Check sheet for the modelled part. Datum: model origin and axes. Units: mm. A direction names the side the tool comes from. Round coordinates to 2 decimals unless told otherwise and drop trailing zeros. Loops run counter-clockwise (first coordinate to the right, second up) from the corner with the lowest first, then second, coordinate; pieces in that order, holes last. Notation, with made-up numbers: (25.5, 3.5) - (49.5, 3.5) arc R19 cw to (49.5, 31.5) - close; hole circle Ø9 at (54.25, 19). An arc over 180 degrees is marked (long way). Put each result on its own line as item: value. Start each with the question number.
```python
from build123d import *

# Parameters (mm, degrees)
BOX001_W          = 50
BOX001_H          = 44
BOX001_DEPTH      = 12.7
CYLINDER001_R     = 6.223
CYLINDER001_DEPTH = 19.05
CYLINDER_R        = 3.175
CYLINDER_DEPTH    = 25.4
CYLINDER003_R     = 6.223
CYLINDER003_DEPTH = 19.05
CYLINDER002_R     = 3.175
CYLINDER002_DEPTH = 25.4
CYLINDER005_R     = 6.223
CYLINDER005_DEPTH = 19.05
CYLINDER004_R     = 3.175
CYLINDER004_DEPTH = 25.4
BOX_W             = 50
BOX_H             = 44
BOX_DEPTH         = 12.7


with BuildPart() as top_plate:
    # Box001 → Box001 (new body)
    with BuildSketch(Plane.XY.offset(21)):
        with Locations((25, 22)):
            Rectangle(BOX001_W, BOX001_H)
    extrude(amount=BOX001_DEPTH)


with BuildPart() as screw_cap:
    # Cylinder001 → Cylinder001 (new body)
    with BuildSketch(Plane.XY.offset(25.4)):
        Circle(CYLINDER001_R)
    extrude(amount=CYLINDER001_DEPTH)


with BuildPart() as left_screw:
    # Cylinder → Cylinder (new body)
    with BuildSketch(Plane.XY):
        Circle(CYLINDER_R)
    extrude(amount=CYLINDER_DEPTH)

    # Fusion: union Screw Cap
    add(screw_cap.part)


with BuildPart() as left_screw_1:
    # Fusion placement: moved
    add(left_screw.part.moved(Location((11, 5.5, 12.7))))


with BuildPart() as screw_cap001:
    # Cylinder003 → Cylinder003 (new body)
    with BuildSketch(Plane.XY.offset(25.4)):
        Circle(CYLINDER003_R)
    extrude(amount=CYLINDER003_DEPTH)


with BuildPart() as right_screw:
    # Cylinder002 → Cylinder002 (new body)
    with BuildSketch(Plane.XY):
        Circle(CYLINDER002_R)
    extrude(amount=CYLINDER002_DEPTH)

    # Fusion001: union Screw Cap001
    add(screw_cap001.part)


with BuildPart() as right_screw_1:
    # Fusion001 placement: moved
    add(right_screw.part.moved(Location((11, 38.5, 12.7))))


with BuildPart() as screw_cap002:
    # Cylinder005 → Cylinder005 (new body)
    with BuildSketch(Plane.XY.offset(25.4)):
        Circle(CYLINDER005_R)
    extrude(amount=CYLINDER005_DEPTH)


with BuildPart() as center_screw:
    # Cylinder004 → Cylinder004 (new body)
    with BuildSketch(Plane.XY):
        Circle(CYLINDER004_R)
    extrude(amount=CYLINDER004_DEPTH)

    # Fusion002: union Screw Cap002
    add(screw_cap002.part)


with BuildPart() as center_screw_1:
    # Fusion002 placement: moved
    add(center_screw.part.moved(Location((44.5, 22, 12.7))))


with BuildPart() as fusion003:
    # Box → Box (new body)
    with BuildSketch(Plane.XY):
        with Locations((25, 22)):
            Rectangle(BOX_W, BOX_H)
    extrude(amount=BOX_DEPTH)

    # Fusion003: union Top Plate, Left Screw, Right Screw, Center Screw
    add(top_plate.part)
    add(left_screw_1.part)
    add(right_screw_1.part)
    add(center_screw_1.part)


solid = fusion003.part
```
Q1. Set-up check for faces 1 (the face through (14.345, 43.747, 47.492)), 2 (the face through (44, 22, 57.15)), 3 (the face through (8, 40, 38.1)): record each of +Z, -Z, +X, -X, +Y, -Y from which the full face is reachable in a straight line by a thin tool's end or side.
Q2. Depth check by flat-ended pin: pin 1 Ø6.5 at (x, z) = (24, 26.5) entering from -Y; pin 2 Ø6.5 at (y, z) = (22.5, 7.5) entering from +X; pin 3 Ø13 at (x, y) = (21, 14) entering from +Z. Enter the tip coordinate at first touch or a pass-through.
Q3. Cross-section at C-C on y = 33.5. Enter the section's corners in (x, z).
Q4. Draft check along Z on faces 4 (the face through (25, 22, 0)), 5 (the face through (14.03, 6.45, 35.87)), 6 (the face through (0, 22, 6)). Enter one of: +Z half, -Z half, draft (parallel to the pull), parting line (faces both ways), or undercut.
Q5. Cross-section at A-A on x = 23. Enter the section's corners in (y, z), and give its area (3 significant figures).
Q6. Material ranges on line 1 (Z direction, x = 8, y = 41); line 2 (Z direction, x = 35, y = 23.5); line 3 (Y direction, x = 36.5, z = 6), recorded low to high. Write a range as from..to.
Q7. Cross-section at D-D on y = 5.5. Enter the section's corners in (x, z) (3 decimals).
Answer list:
1. face 1: +Z
1. face 2: +Z, +X, -X, +Y, -Y
1. face 3: none
2. pin 1: stops at y = 0
2. pin 2: stops at x = 50
2. pin 3: stops at z = 33.7
3. outline: (0, 0) - (50, 0) - (50, 12.7) - (0, 12.7) - close; (0, 21) - (50, 21) - (50, 33.7) - (0, 33.7) - close; (7.3, 38.1) - (14.7, 38.1) - (14.7, 57.15) - (7.3, 57.15) - close
4. face 4: -Z half
4. face 5: undercut
4. face 6: draft
5. outline: (0, 0) - (44, 0) - (44, 12.7) - (0, 12.7) - close; (0, 21) - (44, 21) - (44, 33.7) - (0, 33.7) - close
5. area: 1,120 mm2
6. line 1: z = 0..12.7, 21..33.7, 38.1..57.15
6. line 2: z = 0..12.7, 21..33.7
6. line 3: y = 0..44
7. outline: (0, 0) - (50, 0) - (50, 12.7) - (14.175, 12.7) - (14.175, 21) - (50, 21) - (50, 33.7) - (14.175, 33.7) - (14.175, 38.1) - (17.223, 38.1) - (17.223, 57.15) - (4.777, 57.15) - (4.777, 38.1) - (7.825, 38.1) - (7.825, 33.7) - (0, 33.7) - (0, 21) - (7.825, 21) - (7.825, 12.7) - (0, 12.7) - close
